Input: part model. Units: mm. Frame: model coordinates. A direction names the side the tool comes from. Coordinates: 2 decimals unless noted, no trailing zeros. Order: outer loops, then holes, each group sorted by start corner. A loop starts at its lowest first (then second) coordinate and runs counter-clockwise, first axis right, second up. Notation, with made-up numbers: (-38, 9) -> (9, 9) arc R24 ccw to (9, 42) -> close; hole circle Ø3 at (71, -7.75). An arc over 180 degrees is marked (long way). One line per item, written item: value. Start each with the question number.
Autodesk Inventor part; units mm, degrees
ref_plane "YZ Plane" through (0, 0, 0) normal (1, 0, 0) x (0, 1, 0)
ref_plane "XZ Plane" through (0, 0, 0) normal (0, 1, 0) x (-1, 0, 0)
ref_plane "XY Plane" through (0, 0, 0) normal (0, 0, 1) x (1, 0, 0)
sketch "Sketch1" plane through (0, 0, 0) normal (0, 0, 1) x (1, 0, 0)
  circle A0 centre (0, 0) radius 29.972
  circle A1 centre (0, 0) radius 35.052
  dimension "d0" = 59.944
  dimension "d1" = 5.08
extrude "Extrusion1" add sketch "Sketch1" along normal blind 60.325
sketch "Sketch3" plane through (0, 0, 60.325) normal (0, 0, 1) x (1, 0, 0)
  circle A0 centre (0, 0) radius 29.972
  circle A1 centre (0, 0) radius 35.052
  circle A2 centre (0, 0) radius 30.353
  dimension "d4" = 60.706
extrude "Extrusion2" cut sketch "Sketch3" against normal blind 29.3624 contours A2
sketch "Sketch4" plane through (0, 0, 0) normal (0, 0, -1) x (-1, 0, 0)
  circle A0 centre (0, 0) radius 29.972
  circle A1 centre (0, 0) radius 35.052
  circle A2 centre (0, 0) radius 30.353
  dimension "d7" = 60.706
extrude "Extrusion3" cut sketch "Sketch4" against normal blind 29.3624 contours A2
properties part number "coupler_2in" material "PVC-Piping"
1) Mould query, pull axis Y, two halves, no side actions, for faces 1 (the flat face through (-11, 29, 0)), 2 (the cylindrical face through (33.433, -10.529, 29.74)), 3 (the cylindrical face through (-28.95, 9.12, 14.48)). Classes: +Y half, -Y half, draft (parallel to the pull), parting line (faces both ways), or undercut.
2) Section query A-A, the plane x = 0. Return the cut outline in (y, z) (3 decimals).
3) Pin query (flat end, axial travel): pin 1 Ø5 at (y, z) = (25.5, 32.5) entering from +X; pin 2 Ø5 at (x, z) = (-13, 18) entering from -Y; pin 3 Ø12 at (x, z) = (17, 45.5) entering from +Y; pin 4 Ø18 at (x, y) = (14.5, 11.5) entering from -Z. Return the tip coordinate at first contact, or that it passes through.
4) Access query for faces 4 (the flat face through (-11, 29, 60.325)), 5 (the cylindrical face through (28.95, 9.12, 45.85)). Directions: +Z, -Z, +X, -X, +Y, -Y. A direction counts if a zero-diameter tool reaches every point of the face in a straight line with its end or side. Return the directions, or none.
5) Ray query, line 1 along Y through (x, z) = (0, 18.5); line 2 along Y through (x, z) = (0, 29.9); line 3 along X through (y, z) = (-18, 50). Return the intervals inside material, ascending. Write a range as from..to.
6) Section query C-C, the plane z = 18. Return the cut outline in (x, y), plus the area to 3 significant figures.
Entries:
1. face 1: draft
1. face 2: parting line
1. face 3: undercut
2. outline: (-35.052, 0) -> (-30.353, 0) -> (-30.353, 29.362) -> (-29.972, 29.362) -> (-29.972, 30.963) -> (-30.353, 30.963) -> (-30.353, 60.325) -> (-35.052, 60.325) -> close; (29.972, 29.362) -> (30.353, 29.362) -> (30.353, 0) -> (35.052, 0) -> (35.052, 60.325) -> (30.353, 60.325) -> (30.353, 30.963) -> (29.972, 30.963) -> close
3. pin 1: stops at x = 26.45
3. pin 2: stops at y = -33.44
3. pin 3: stops at y = 33.28
3. pin 4: passes through
4. face 4: +Z, +X, -X, +Y, -Y
4. face 5: +Z
5. line 1: y = -35.05..-30.35, 30.35..35.05
5. line 2: y = -35.05..-29.97, 29.97..35.05
5. line 3: x = -30.08..-24.44, 24.44..30.08
6. outline: circle Ø70.1 at (0, 0); hole circle Ø60.71 at (0, 0)
6. area: 966 mm2
